from build123d import *

# Parameters (mm, degrees)
F0_R     = 4
F1_DEPTH = 5
F2_R     = 2.5
F3_DEPTH = 25
F6_W     = 1.75
F6_H     = 1.5
F6_W_2   = 1.5
F6_H_2   = 1.75
F7_DEPTH = 3
F9_ANGLE = 180


with BuildPart() as f1:
    # F0 (on Top) → F1 (new body)
    with BuildSketch(Plane.XY):
        Circle(F0_R)
    extrude(amount=F1_DEPTH)

    # F2 (on face) → F3 (join)
    with BuildSketch(Plane.XY.offset(5)):
        Circle(F2_R)
    extrude(amount=F3_DEPTH)

    # F4 (on Front) → F5 (revolve, cut)
    with BuildSketch(Plane.XZ):
        Polygon((-4, 0.5), (-2.5, 5), (-4, 5), align=None)
    revolve(axis=Axis((0, 0, 2.5), (0, 0, -1)), mode=Mode.SUBTRACT)

    # F6 (on face) → F7 (cut)
    with BuildSketch(Plane(origin=(0, 0, 0), x_dir=(1, 0, 0), z_dir=(0, 0, -1))):
        with Locations((1.625, 0)):
            Rectangle(F6_W, F6_H)
        Rectangle(F6_W_2, F6_H)
        with Locations((0, 1.625)):
            Rectangle(F6_W_2, F6_H_2)
        with Locations((-1.625, 0)):
            Rectangle(F6_W, F6_H)
        with Locations((0, -1.625)):
            Rectangle(F6_W_2, F6_H_2)
    extrude(amount=-F7_DEPTH, mode=Mode.SUBTRACT)


with BuildPart() as f1_1:
    # F9: moved
    add(f1.part.rotate(Axis((9.6651110798, 0, 0), (1, 0, 0)), F9_ANGLE))


solid = f1_1.part
Model file for the job. Use its own axes, mm. A direction names the side the tool comes from. Give positions to 0.01 mm unless a question says otherwise; leave off trailing zeros. Write each loop counter-clockwise with the first axis right and the second up, starting at its lowest first coordinate (ties: lowest second). Pieces come first, ordered by that corner, then holes. Notation, with made-up numbers: (5.5, 37) -> (53.5, 37) arc R13 cw to (53.5, 57) -> close; hole circle Ø10 at (3.5, 35). An arc over 180 degrees is marked (long way). Write item = value, one per line.
(1) Slice it at A-A, the plane x = 0. Give the cut face in (y, z).
Determined:
outline = (-4, -0.5) -> (-2.5, -5) -> (-2.5, -30) -> (2.5, -30) -> (2.5, -5) -> (4, -0.5) -> (4, 0) -> (2.5, 0) -> (2.5, -3) -> (-2.5, -3) -> (-2.5, 0) -> (-4, 0) -> close
(2) Probe line 1 along Z through (x, y) = (0, -1); line 2 along X through (y, z) = (0, -2); line 3 along Y through (x, z) = (2.25, -16.75). List the from-to ranges inside material, lowest first.
Determined:
line_1 = -30 to -3
line_2 = -3.5 to -2.5, 2.5 to 3.5
line_3 = -1.09 to 1.09
(3) Flat gauge pins, fed straight in: P1, Ø1, axis at x = 2.5, z = -18.5, coming from the +Y side; P2, Ø0.8, axis at y = 0, z = -2, coming from the -X side; P3, Ø1.4, axis at x = -2, z = -1, coming from the +Y side. Where does each tip first touch, or does it go through?
Determined:
P1 = 1.5
P2 = -3.63
P3 = 3.7
(4) Mould opens along Y. For faces 4 (the face through (0.75, 2, -1)), 5 (the face through (1, 1, 0)), 6 (the face through (2.306, 1.768, -3.782)) say: released by +Y, released by -Y, zero draft, split by the parting line, or undercut.
Determined:
face_4 = undercut
face_5 = zero draft
face_6 = split by the parting line
(5) Slice it at C-C, the plane z = -5.5. Give the cut face in (x, y), then the cut area to 3 significant figures.
Determined:
outline = circle Ø5 at (0, 0)
area = 19.6 mm2
(6) Tool access for faces 1 (the face through (-0.867, 3.905, -0.247)), 2 (the face through (-2.5, -0.1, -17.3)), 3 (the face through (2, 0.75, -1)): list every direction of +Z, -Z, +X, -X, +Y, -Y with a clear straight run to the whole face (end or side of a thin tool).
Determined:
face_1 = +Z, -Z
face_2 = -Z
face_3 = +Z
